from build123d import *

# Parameters (mm, degrees)
SKETCH1_R           = 4
SKETCH1_R_2         = 3
BOSS_EXTRUDE1_DEPTH = 4
SKETCH2_R           = 6
SKETCH2_R_2         = 3
BOSS_EXTRUDE2_DEPTH = 1
FILLET1_R           = 0.5
CHAMFER1_SIZE       = 0.3
CHAMFER1_SIZE2      = 0.173205081


with BuildPart() as part:
    # Sketch1 → Boss-Extrude1 (new body)
    with BuildSketch(Plane.XY):
        Circle(SKETCH1_R)
        Circle(SKETCH1_R_2, mode=Mode.SUBTRACT)
    extrude(amount=BOSS_EXTRUDE1_DEPTH)

    # Sketch2 → Boss-Extrude2 (add)
    with BuildSketch(Plane.XY.offset(4)):
        Circle(SKETCH2_R)
        Circle(SKETCH2_R_2, mode=Mode.SUBTRACT)
    extrude(amount=-BOSS_EXTRUDE2_DEPTH)

    # Fillet1
    fillet1_edges = [part.edges().sort_by_distance(p)[0] for p in [
        (-4, 0, 3),
    ]]
    fillet(fillet1_edges, radius=FILLET1_R)

    # Chamfer1
    chamfer1_edges = [part.edges().sort_by_distance(p)[0] for p in [
        (-4, 0, 0),
    ]]
    chamfer1_side = [part.faces().sort_by_distance(p)[0] for p in [
        (-4, 0, 1.25),
    ]]
    chamfer(chamfer1_edges, length=CHAMFER1_SIZE, length2=CHAMFER1_SIZE2, reference=chamfer1_side[0])


solid = part.part
Could you check a few things on this model? Use its own coordinates, in mm. A direction names the side the tool comes from. Give positions to 0.01 mm unless a question says otherwise; leave off trailing zeros. Loops run counter-clockwise (first coordinate to the right, second up) from the corner with the lowest first, then second, coordinate; pieces in that order, holes last. Notation, with made-up numbers: (79, 71.5) -> (130, 71.5) arc R20 ccw to (130, 77.5) -> close; hole circle Ø2 at (13.5, 19). An arc over 180 degrees is marked (long way). Answer as CSV lines item,"result". Start each with the question number.
(1) I need wall thicknesses on probe 1 along Y at (x, z) = (0, 2.1); probe 2 along Z at (x, y) = (3.75, -4.5); probe 3 along X at (y, z) = (2, 2.1). Which ranges of each line are inside material? Lowest first, please.
(2) If we section it at D-D on x = 5.75: Write out the boundary of the cut face in (y, z).
(3) We'd pull the mould along Y, two halves only. Please class faces 1 (the cylindrical face through (-0.867, -3.905, 1.385)), 2 (the flat face through (2, -3, 0)), 3 (the cylindrical face through (-3, 0, 2)): released by +Y, released by -Y, zero draft, split by the parting line, or undercut.
(4) Which directions (+Z, -Z, +X, -X, +Y, -Y) give clear straight access to the entire face, cutting with the end or side of a thin tool? Please do faces 4 (the flat face through (-1.4, 4.5, 3)), 5 (the cylindrical face through (-5.994, 0.264, 3.507)).
(5) If we section it at A-A on y = 0: Write out the boundary of the cut face in (x, z), then the cut area to 3 significant figures.
(6) If we section it at C-C on z = 0.45: Write out the boundary of the cut face in (x, y), then the cut area to 3 significant figures.
Computed:
1,probe 1,"y = -4 to -3, 3 to 4"
1,probe 2,"z = 3 to 4"
1,probe 3,"x = -3.46 to -2.24, 2.24 to 3.46"
2,outline,"(-1.71, 3) -> (1.71, 3) -> (1.71, 4) -> (-1.71, 4) -> close"
3,face 1,"split by the parting line"
3,face 2,"zero draft"
3,face 3,"undercut"
4,face 4,"-Z"
4,face 5,"+Z, -Z"
5,outline,"(-6, 3) -> (-4.5, 3) arc R0.5 cw to (-4, 2.5) -> (-4, 0.3) -> (-3.83, 0) -> (-3, 0) -> (-3, 4) -> (-6, 4) -> close; (3, 0) -> (3.83, 0) -> (4, 0.3) -> (4, 2.5) arc R0.5 cw to (4.5, 3) -> (6, 3) -> (6, 4) -> (3, 4) -> close"
5,area,"12.1 mm2"
6,outline,"circle Ø8 at (0, 0); hole circle Ø6 at (0, 0)"
6,area,"22.0 mm2"
